Part model, mm, in its own coordinate system. A direction names the side the tool comes from. Coordinates: 2 decimals unless noted, no trailing zeros. Order: outer loops, then holes, each group sorted by start corner. A loop starts at its lowest first (then second) coordinate and runs counter-clockwise, first axis right, second up.
```python
from build123d import *

# Parameters (mm, degrees)
SKETCH_1_R          = 2.5
SKETCH_1_R_2        = 2.45
SKETCH_1_R_3        = 1.85
SKETCH_1_W          = 48
SKETCH_1_H          = 40
EXTRUDE_1_DEPTH     = 3
CUT_EXTRUDE_1_REACH = 82.678
SKETCH_2_W          = 40
SKETCH_2_H          = 50
SKETCH_3_R          = 2.65
CUT_EXTRUDE_2_DEPTH = 10


with BuildPart() as part:
    # 草图1 → 凸台-拉伸1 (new body)
    # profile 1 of 5: a face of its own
    with BuildSketch(Plane(origin=(0, 0, 0), x_dir=(1, 0, 0), z_dir=(0, 1, 0))):
        with BuildLine():
            Line((8, -30), (8, -70))
            Line((8, -70), (40, -70))
            Line((40, -70), (40, 60))
            Line((40, 60), (32.5, 60))
            ThreePointArc((32.5, 60), (28.232233047, 58.232233047), (30, 62.5))
            Line((30, 62.5), (30, 70))
            Line((30, 70), (8, 70))
            Line((8, 70), (8, 30))
            Line((8, 30), (-40, 30))
            Line((-40, 30), (-40, -30))
            Line((-40, -30), (8, -30))
        make_face()
        with Locations(Location((30, -60, 0), (0, 0, 270))):
            Circle(SKETCH_1_R, mode=Mode.SUBTRACT)
        with Locations(Location((30, 0, 0), (0, 0, 270))):
            Circle(SKETCH_1_R, mode=Mode.SUBTRACT)
    # profile 2 of 5: a face of its own
    with BuildSketch(Plane(origin=(0, 0, 0), x_dir=(1, 0, 0), z_dir=(0, 1, 0))):
        with BuildLine():
            Line((32.5, 60), (40, 60))
            Line((40, 60), (40, 70))
            Line((40, 70), (30, 70))
            Line((30, 70), (30, 62.5))
            ThreePointArc((30, 62.5), (31.767766953, 61.767766953), (32.5, 60))
        make_face()
    # profile 3 of 5: a face of its own
    with BuildSketch(Plane(origin=(0, 0, 0), x_dir=(1, 0, 0), z_dir=(0, 1, 0))):
        with BuildLine():
            Line((-40, 61.45), (-40, 30))
            Line((-40, 30), (8, 30))
            Line((8, 30), (8, 70))
            Line((8, 70), (-30, 70))
            Line((-30, 70), (-30, 63.3))
            ThreePointArc((-30, 63.3), (-28.691852455, 62.758147545), (-28.15, 61.45))
            ThreePointArc((-28.15, 61.45), (-30, 59.6), (-31.85, 61.45))
            Line((-31.85, 61.45), (-40, 61.45))
        make_face()
        with Locations(Location((-31.5, 50, 0), (0, 0, 270))):
            Circle(SKETCH_1_R_2, mode=Mode.SUBTRACT)
        with Locations(Location((-30, 38.55, 0), (0, 0, 270))):
            Circle(SKETCH_1_R_3, mode=Mode.SUBTRACT)
        with Locations(Location((-2, 38.55, 0), (0, 0, 270))):
            Circle(SKETCH_1_R_3, mode=Mode.SUBTRACT)
        with Locations(Location((-0.5, 50, 0), (0, 0, 270))):
            Circle(SKETCH_1_R_2, mode=Mode.SUBTRACT)
        with Locations(Location((-2, 61.45, 0), (0, 0, 270))):
            Circle(SKETCH_1_R_3, mode=Mode.SUBTRACT)
    # profile 4 of 5: a face of its own
    with BuildSketch(Plane(origin=(0, 0, 0), x_dir=(1, 0, 0), z_dir=(0, 1, 0))):
        with BuildLine():
            Line((-40, 70), (-40, 61.45))
            Line((-40, 61.45), (-31.85, 61.45))
            ThreePointArc((-31.85, 61.45), (-31.308147545, 62.758147545), (-30, 63.3))
            Line((-30, 63.3), (-30, 70))
            Line((-30, 70), (-40, 70))
        make_face()
    # profile 5 of 5: a face of its own
    with BuildSketch(Plane(origin=(0, 0, 0), x_dir=(1, 0, 0), z_dir=(0, 1, 0))):
        with Locations((-16, -50)):
            Rectangle(SKETCH_1_W, SKETCH_1_H)
        with Locations(Location((-30, -61.45, 0), (0, 0, 270))):
            Circle(SKETCH_1_R_3, mode=Mode.SUBTRACT)
        with Locations(Location((-31.5, -50, 0), (0, 0, 270))):
            Circle(SKETCH_1_R_2, mode=Mode.SUBTRACT)
        with Locations(Location((-30, -38.55, 0), (0, 0, 270))):
            Circle(SKETCH_1_R_3, mode=Mode.SUBTRACT)
        with Locations(Location((-2, -61.45, 0), (0, 0, 270))):
            Circle(SKETCH_1_R_3, mode=Mode.SUBTRACT)
        with Locations(Location((-0.5, -50, 0), (0, 0, 270))):
            Circle(SKETCH_1_R_2, mode=Mode.SUBTRACT)
        with Locations(Location((-2, -38.55, 0), (0, 0, 270))):
            Circle(SKETCH_1_R_3, mode=Mode.SUBTRACT)
    extrude(amount=EXTRUDE_1_DEPTH)

    # 草图2 → 切除-拉伸1 (cut, up to next)
    with BuildSketch(Plane(origin=(0, 3, 0), x_dir=(1, 0, 0), z_dir=(0, 1, 0)), mode=Mode.PRIVATE) as cut_extrude_1_sk1:
        Rectangle(SKETCH_2_W, SKETCH_2_H)
    cut_extrude_1_tool1 = extrude(cut_extrude_1_sk1.sketch, amount=-CUT_EXTRUDE_1_REACH, mode=Mode.PRIVATE) & part.part
    add(cut_extrude_1_tool1.solids().sort_by_distance((0, 3, 0))[0], mode=Mode.SUBTRACT)

    # 草图3 → 切除-拉伸2 (cut)
    with BuildSketch(Plane(origin=(0, 3, 0), x_dir=(1, 0, 0), z_dir=(0, 1, 0))):
        with Locations(Location((30, 60, 0), (0, 0, 270))):
            Circle(SKETCH_3_R)
        with Locations(Location((30, 0, 0), (0, 0, 270))):
            Circle(SKETCH_3_R)
        with Locations(Location((30, -60, 0), (0, 0, 270))):
            Circle(SKETCH_3_R)
    extrude(amount=-CUT_EXTRUDE_2_DEPTH, mode=Mode.SUBTRACT)


solid = part.part
```
(1) Slice it at D-D, the plane z = 50. Give the cut face in (x, y).
(2) Tool access for faces 5 (the face through (0, 2, -25)), 6 (the face through (40, 1, 1)): list every direction of +Z, -Z, +X, -X, +Y, -Y with a clear straight run to the whole face (end or side of a thin tool).
(3) Slice it at C-C, the plane z = -38.55. Give the cut face in (x, y), then the cut area to 3 significant figures.
(4) Pull direction Z, two halves, no side cores. Call faces 1 (the face through (1, 1, -70)), 2 (the face through (-40, 1, 1)), 3 (the face through (-1, 1, 70)), 4 (the face through (-20, 2, 0)): +Z half, -Z half, draft (parallel to the pull), parting line (faces both ways), or undercut.
(5) Probe line 1 (X direction, y = 0.85, z = -50); line 2 (X direction, y = 1.85, z = 0); line 3 (Z direction, x = -13, y = 1.5). List the from-to ranges inside material, lowest first.
(6) Slice it at B-B, the plane z = 21. Give the cut face in (x, y), then the cut area to 3 significant figures.
(7) Drop a flat-ended pin along its axis: pin 1 (6 mm diameter, centred on x = 30, z = 0, fed in from -Y). Give the stop position or say it passes through.
(8) Slice it at A-A, the plane y = 1.4. State how many separate pieces and enclosed holes the cut face has, then the cut area to 3 significant figures.
Here are the results:
1. outline: (-40, 0) - (-33.95, 0) - (-33.95, 3) - (-40, 3) - close; (-29.05, 0) - (-2.95, 0) - (-2.95, 3) - (-29.05, 3) - close; (1.95, 0) - (40, 0) - (40, 3) - (1.95, 3) - close
2. face 5: +Y, -Y
2. face 6: +Z, -Z, +X, +Y, -Y
3. outline: (-40, 0) - (-31.85, 0) - (-31.85, 3) - (-40, 3) - close; (-28.15, 0) - (-3.85, 0) - (-3.85, 3) - (-28.15, 3) - close; (-0.15, 0) - (40, 0) - (40, 3) - (-0.15, 3) - close
3. area: 218 mm2
4. face 1: -Z half
4. face 2: draft
4. face 3: +Z half
4. face 4: undercut
5. line 1: x = -40 to -33.95, -29.05 to -2.95, 1.95 to 40
5. line 2: x = -40 to -20, 20 to 27.35, 32.65 to 40
5. line 3: z = -70 to -25, 25 to 70
6. outline: (-40, 0) - (-20, 0) - (-20, 3) - (-40, 3) - close; (20, 0) - (40, 0) - (40, 3) - (20, 3) - close
6. area: 120 mm2
7. pin 1: stops at y = 0
8. separate pieces: 1
8. enclosed holes: 16
8. area: 8,970 mm2
